from build123d import *

# Parameters (mm, degrees)
SKETCH1_R           = 6
SKETCH1_R_2         = 1
BOSS_EXTRUDE1_DEPTH = 5
FILLET2_R           = 2


with BuildPart() as part:
    # Sketch1 → Boss-Extrude1 (new body)
    with BuildSketch(Plane(origin=(0, 0, 0), x_dir=(1, 0, 0), z_dir=(0, 1, 0))):
        with BuildLine():
            Line((0, 0), (30, 0))
            Line((30, 0), (30, 48))
            Line((30, 48), (0, 48))
            Line((0, 48), (0, 35.5))
            ThreePointArc((0, 35.5), (-2.5, 33), (0, 30.5))
            Line((0, 30.5), (0, 17.5))
            ThreePointArc((0, 17.5), (-2.5, 15), (0, 12.5))
            Line((0, 12.5), (0, 0))
        make_face()
        with Locations(Location((21, 38, 0), (0, 0, 270))):
            Circle(SKETCH1_R, mode=Mode.SUBTRACT)
        with Locations(Location((21, 10, 0), (0, 0, 270))):
            Circle(SKETCH1_R, mode=Mode.SUBTRACT)
        with Locations(Location((0, 33, 0), (0, 0, 270))):
            Circle(SKETCH1_R_2, mode=Mode.SUBTRACT)
        with Locations(Location((0, 15, 0), (0, 0, 270))):
            Circle(SKETCH1_R_2, mode=Mode.SUBTRACT)
    extrude(amount=BOSS_EXTRUDE1_DEPTH)

    # Fillet2
    fillet2_edges = [part.edges().sort_by_distance(p)[0] for p in [
        (30, 2.5, 0),
        (0, 2.5, 0),
        (0, 2.5, -48),
        (30, 2.5, -48),
    ]]
    fillet(fillet2_edges, radius=FILLET2_R)


solid = part.part
Verification items for the finished model (mm, model axes). A direction names the side the tool comes from. Coordinates: 2 decimals unless noted, no trailing zeros. Order: outer loops, then holes, each group sorted by start corner. A loop starts at its lowest first (then second) coordinate and runs counter-clockwise, first axis right, second up.
Item 1: Release check for a two-part mould opening along X. For faces 1 (the face through (-2.5, 2.5, -15.1)), 2 (the face through (0, 2, -14)), 3 (the face through (29.43, 2.54, -47.4)) record: +X half, -X half, draft (parallel to the pull), parting line (faces both ways), or undercut.
Filled in:
face 1: -X half
face 2: undercut
face 3: +X half
Item 2: Section check D-D, the plane z = -33. Enter the section's corners in (x, y).
Filled in:
outline: (-2.5, 0) - (-1, 0) - (-1, 5) - (-2.5, 5) - close; (1, 0) - (17.68, 0) - (17.68, 5) - (1, 5) - close; (24.32, 0) - (30, 0) - (30, 5) - (24.32, 5) - close
Item 3: Material ranges on L1, parallel to X at y = 2.85, z = -33; L2, parallel to X at y = 2.8, z = -10; L3, parallel to X at y = 1.6, z = -22, recorded low to high.
Filled in:
L1: x = -2.5 to -1, 1 to 17.68, 24.32 to 30
L2: x = 0 to 15, 27 to 30
L3: x = 0 to 30
Item 4: Section check B-B, the plane y = 1.3. Enter the section's corners in (x, z).
Filled in:
outline: (0, -46) arc R2 ccw to (2, -48) - (28, -48) arc R2 ccw to (30, -46) - (30, -2) arc R2 ccw to (28, 0) - (2, 0) arc R2 ccw to (0, -2) - (0, -12.5) arc R2.5 ccw to (0, -17.5) - (0, -30.5) arc R2.5 ccw to (0, -35.5) - close; hole circle Ø2 at (0, -33); hole circle Ø2 at (0, -15); hole circle Ø12 at (21, -38); hole circle Ø12 at (21, -10)
Item 5: Depth check by flat-ended pin: pin 1 (1.2 mm diameter, centred on x = 0, z = -33, fed in from +Y); pin 2 (2.5 mm diameter, centred on y = 2.5, z = -5.5, fed in from -X). Enter the tip coordinate at first touch or a pass-through.
Filled in:
pin 1: passes through
pin 2: stops at x = 0
Item 6: Access from +Z, -Z, +X, -X, +Y, -Y to the whole of each face (thin tool, end or side, straight path). Record for faces 4 (the face through (0, 2, -24)), 5 (the face through (0, 2, -7)), 6 (the face through (0, 2, -41)).
Filled in:
face 4: -X, +Y, -Y
face 5: +Z, -X, +Y, -Y
face 6: -Z, -X, +Y, -Y
Item 7: Section check A-A, the plane x = 21. Enter the section's corners in (y, z), then the cut area to 3 significant figures.
Filled in:
outline: (0, -48) - (5, -48) - (5, -44) - (0, -44) - close; (0, -32) - (5, -32) - (5, -16) - (0, -16) - close; (0, -4) - (5, -4) - (5, 0) - (0, 0) - close
area: 120 mm2
Item 8: Section check C-C, the plane z = -10. Enter the section's corners in (x, y), then the cut area to 3 significant figures.
Filled in:
outline: (0, 0) - (15, 0) - (15, 5) - (0, 5) - close; (27, 0) - (30, 0) - (30, 5) - (27, 5) - close
area: 90.0 mm2
